Verification items for the finished model (mm, model axes). A direction names the side the tool comes from. Coordinates: 2 decimals unless noted, no trailing zeros. Order: outer loops, then holes, each group sorted by start corner. A loop starts at its lowest first (then second) coordinate and runs counter-clockwise, first axis right, second up. Notation, with made-up numbers: M 60.5,25.5 L 91.5,25.5 A25 ccw 91.5,54.5 Z; hole C 34,-25.75 d10. An arc over 180 degrees is marked long. Write item = value, one per line.
```python
from build123d import *

# Parameters (mm, degrees)
SKETCH3_R           = 18
BOSS_EXTRUDE1_DEPTH = 1
SKETCH4_R           = 11
CUT_EXTRUDE1_DEPTH  = 1
SKETCH5_R           = 1.15
CUT_EXTRUDE2_DEPTH  = 6
SKETCH6_R           = 11
SKETCH6_R_2         = 1.15
BOSS_EXTRUDE2_DEPTH = 3
SKETCH9_R           = 11
SKETCH9_R_2         = 2.15
BOSS_EXTRUDE3_DEPTH = 2


with BuildPart() as part:
    # Sketch1 → Revolve1 (revolve)
    with BuildSketch(Plane.XY):
        Polygon((18, 5), (18, -5), (19.75, -5), (19.75, -1), (21.75, -1), (21.75, 1), (19.75, 1), (19.75, 5), align=None)
    revolve(axis=Axis((0, 0, 0), (0, 1, 0)))

    # Sketch3 → Boss-Extrude1 (add, symmetric)
    with BuildSketch(Plane(origin=(0, 0, 0), x_dir=(1, 0, 0), z_dir=(0, 1, 0))):
        Circle(SKETCH3_R)
        with BuildLine():
            ThreePointArc((-6.792630924, -16.398861702), (-8.145621175, -13.13245429), (-4.879213763, -11.77946404))
            ThreePointArc((-4.879213763, -11.77946404), (0, -12.75), (4.879213763, -11.77946404))
            ThreePointArc((4.879213763, -11.77946404), (8.145621175, -13.13245429), (6.792630924, -16.398861702))
            ThreePointArc((6.792630924, -16.398861702), (0, -17.75), (-6.792630924, -16.398861702))
        make_face(mode=Mode.SUBTRACT)
        with BuildLine():
            ThreePointArc((16.398861702, -6.792630924), (13.13245429, -8.145621175), (11.77946404, -4.879213763))
            ThreePointArc((11.77946404, -4.879213763), (12.75, 0), (11.77946404, 4.879213763))
            ThreePointArc((11.77946404, 4.879213763), (13.13245429, 8.145621175), (16.398861702, 6.792630924))
            ThreePointArc((16.398861702, 6.792630924), (17.75, 0), (16.398861702, -6.792630924))
        make_face(mode=Mode.SUBTRACT)
        with BuildLine():
            ThreePointArc((-16.398861702, 6.792630924), (-13.13245429, 8.145621175), (-11.77946404, 4.879213763))
            ThreePointArc((-11.77946404, 4.879213763), (-12.75, 0), (-11.77946404, -4.879213763))
            ThreePointArc((-11.77946404, -4.879213763), (-13.13245429, -8.145621175), (-16.398861702, -6.792630924))
            ThreePointArc((-16.398861702, -6.792630924), (-17.75, 0), (-16.398861702, 6.792630924))
        make_face(mode=Mode.SUBTRACT)
        with BuildLine():
            ThreePointArc((-4.879213763, 11.77946404), (-8.145621175, 13.13245429), (-6.792630924, 16.398861702))
            ThreePointArc((-6.792630924, 16.398861702), (0, 17.75), (6.792630924, 16.398861702))
            ThreePointArc((6.792630924, 16.398861702), (8.145621175, 13.13245429), (4.879213763, 11.77946404))
            ThreePointArc((4.879213763, 11.77946404), (0, 12.75), (-4.879213763, 11.77946404))
        make_face(mode=Mode.SUBTRACT)
    extrude(amount=BOSS_EXTRUDE1_DEPTH, both=True)

    # Sketch4 → Cut-Extrude1 (cut)
    with BuildSketch(Plane(origin=(0, 1, 0), x_dir=(1, 0, 0), z_dir=(0, 1, 0))):
        Circle(SKETCH4_R)
    extrude(amount=-CUT_EXTRUDE1_DEPTH, mode=Mode.SUBTRACT)

    # Sketch5 → Cut-Extrude2 (cut, through all)
    with BuildSketch(Plane(origin=(0, 0, 0), x_dir=(1, 0, 0), z_dir=(0, 1, 0))):
        with Locations((0, -8)):
            Circle(SKETCH5_R)
        with Locations((-6.92820323, 4)):
            Circle(SKETCH5_R)
        with Locations((6.92820323, 4)):
            Circle(SKETCH5_R)
        Polygon((3.175426481, 0), (1.58771324, 2.75), (-1.58771324, 2.75), (-3.175426481, 0), (-1.58771324, -2.75), (1.58771324, -2.75), align=None)
    extrude(amount=-CUT_EXTRUDE2_DEPTH, mode=Mode.SUBTRACT)

    # Sketch6 → Boss-Extrude2 (add)
    with BuildSketch(Plane.XZ.offset(1)):
        Circle(SKETCH6_R)
        with Locations((-6.92820323, -4)):
            Circle(SKETCH6_R_2, mode=Mode.SUBTRACT)
        with Locations((6.92820323, -4)):
            Circle(SKETCH6_R_2, mode=Mode.SUBTRACT)
        with Locations((0, 8)):
            Circle(SKETCH6_R_2, mode=Mode.SUBTRACT)
        Polygon((3.175426481, 0), (1.58771324, -2.75), (-1.58771324, -2.75), (-3.175426481, 0), (-1.58771324, 2.75), (1.58771324, 2.75), align=None, mode=Mode.SUBTRACT)
    extrude(amount=BOSS_EXTRUDE2_DEPTH)

    # Sketch9 → Boss-Extrude3 (add)
    with BuildSketch(Plane.XZ.offset(4)):
        Circle(SKETCH9_R)
        with Locations((0, 8)):
            Circle(SKETCH9_R_2, mode=Mode.SUBTRACT)
        with Locations((-6.92820323, -4)):
            Circle(SKETCH9_R_2, mode=Mode.SUBTRACT)
        with Locations((6.92820323, -4)):
            Circle(SKETCH9_R_2, mode=Mode.SUBTRACT)
        Polygon((-1.58771324, -2.75), (1.58771324, -2.75), (3.175426481, 0), (1.58771324, 2.75), (-1.58771324, 2.75), (-3.175426481, 0), align=None, mode=Mode.SUBTRACT)
    extrude(amount=BOSS_EXTRUDE3_DEPTH)


solid = part.part
```
Item 1: Gauge pin test, flat ends, axial feed: pin 1 (1.5 mm diameter, centred on x = 17, y = -3.5, fed in from +Z) (3 decimals); pin 2 (4 mm diameter, centred on x = -6.93, z = -4, fed in from -Y); pin 3 (10 mm diameter, centred on x = 5, z = -1, fed in from +Y). Record the tip position at first contact, or that the pin passes through.
Report:
pin_1 = 11.225
pin_2 = -4
pin_3 = 0
Item 2: Scan lines: L1, parallel to Z at x = 0, y = -2.6; L2, parallel to Z at x = 0, y = -4.5; L3, parallel to X at y = 0.3, z = 0. Record each from-to range of solid material in increasing order. Write a range as from..to.
Report:
L1 = -19.75..-18, -11..-2.75, 2.75..6.85, 9.15..11, 18..19.75
L2 = -19.75..-18, -11..-2.75, 2.75..5.85, 10.15..11, 18..19.75
L3 = -21.75..-17.75, -12.75..-11, 11..12.75, 17.75..21.75
Item 3: Sectioned sample at D-D, the plane x = 0. Give the number of separate pieces and of enclosed holes in the cut face, then the cut area to 3 significant figures.
Report:
separate_pieces = 5
enclosed_holes = 0
area = 132 mm^2
Item 4: Sectioned sample at C-C, the plane z = 15. Enter the section's corners in (x, y), then the cut area to 3 significant figures.
Report:
outline = M -15.75,-1 L -12.85,-1 L -12.85,-5 L -9.95,-5 L -9.95,-1 L -8.16,-1 L -8.16,1 L -9.95,1 L -9.95,5 L -12.85,5 L -12.85,1 L -15.75,1 Z; M 8.16,-1 L 9.95,-1 L 9.95,-5 L 12.85,-5 L 12.85,-1 L 15.75,-1 L 15.75,1 L 12.85,1 L 12.85,5 L 9.95,5 L 9.95,1 L 8.16,1 Z
area = 76.7 mm^2
Item 5: Sectioned sample at B-B, the plane x = -15.5. Enter the section's corners in (y, z), then the cut area to 3 significant figures.
Report:
outline = M -5,-12.24 L -1,-12.24 L -1,-15.26 L 1,-15.26 L 1,-12.24 L 5,-12.24 L 5,-9.15 L 1,-9.15 L 1,-7.9 L -1,-7.9 L -1,-9.15 L -5,-9.15 Z; M -5,9.15 L -1,9.15 L -1,7.9 L 1,7.9 L 1,9.15 L 5,9.15 L 5,12.24 L 1,12.24 L 1,15.26 L -1,15.26 L -1,12.24 L -5,12.24 Z
area = 78.8 mm^2
Item 6: Tool access check on faces 1 (the flat face through (9, 5, 16)), 2 (the cylindrical face through (-2.38, 0.51, 10.74)), 3 (the cylindrical face through (-0.28, -4.99, 10.13)), 4 (the cylindrical face through (0.07, 0.01, -12.75)). Record the directions out of +Z, -Z, +X, -X, +Y, -Y that give a thin tool (end or side, any length) a straight path to the whole face; none if there is none.
Report:
face_1 = +Z, -Z, +X, -X, +Y
face_2 = +Y
face_3 = -Y
face_4 = +Y, -Y
Item 7: Release check for a two-part mould opening along X. For faces 5 (the flat face through (1, -4, 7)), 6 (the flat face through (-9, -5, 16)), 7 (the cylindrical face through (-2.831, 0.014, -21.565)) record: pulls with the +X half, pulls with the -X half, needs draft (parallel to the pull), parting line crosses it, or undercut.
Report:
face_5 = undercut
face_6 = needs draft
face_7 = parting line crosses it
Item 8: Sectioned sample at A-A, the plane y = -3. Enter the section's corners in (x, z).
Report:
outline = C 0,0 d39.5; C 0,0 d22; hole C 0,0 d36; hole C -6.93,-4 d2.3; hole M -3.18,0 L -1.59,-2.75 L 1.59,-2.75 L 3.18,0 L 1.59,2.75 L -1.59,2.75 Z; hole C 0,8 d2.3; hole C 6.93,-4 d2.3
